from build123d import *

# Parameters (mm, degrees)
SKETCH1_W             = 89.6514
SKETCH1_H             = 226.9314
SKETCH1_R             = 2
HEAT_EXCHANGER_DEPTH  = 0.0686
CONVECTION_FINS_DEPTH = 7.0524
TOP_OVERWRAP_DEPTH    = 0.0686
SIDE_OVERWRAP_DEPTH   = 0.0686


# Read off the part's stored shape, not the designer's step: Mirror1
with BuildPart() as part:
    # Sketch1 → Heat Exchanger (new body)
    with BuildSketch(Plane.XY):
        with Locations((-44.8257, 0)):
            Rectangle(SKETCH1_W, SKETCH1_H)
        with Locations((-83.71996294, -56.7081132)):
            Circle(SKETCH1_R, mode=Mode.SUBTRACT)
        with Locations((-83.71996294, 56.94427919)):
            Circle(SKETCH1_R, mode=Mode.SUBTRACT)
    extrude(amount=HEAT_EXCHANGER_DEPTH)

    # Sketch3 → Convection Fins (add)
    with BuildSketch(Plane.XY):
        Polygon((0, -113.5343), (0, -113.4657), (-89.6514, -113.4657), (-89.6514, 113.4657), (-89.72, 113.4657), (-89.72, -113.5343), align=None)
    extrude(amount=CONVECTION_FINS_DEPTH)

    # Sketch5 → Top Overwrap (add)
    with BuildSketch(Plane(origin=(0, 113.4657, 0), x_dir=(1, 0, 0), z_dir=(0, 1, 0))):
        Polygon((-89.8724, -7.0524), (-89.6514, -7.0524), (-89.6514, -0.0686), (0, -0.0686), (0, 0.1524), (-89.8724, 0.1524), align=None)
    extrude(amount=TOP_OVERWRAP_DEPTH)

    # Sketch7 → Side Overwrap (add)
    with BuildSketch(Plane.XY.offset(7.0524)):
        Polygon((-89.8724, 113.5343), (-89.6514, 113.5343), (-89.6514, -113.4657), (0, -113.4657), (0, -113.6867), (-89.8724, -113.6867), align=None)
    extrude(amount=SIDE_OVERWRAP_DEPTH)

    # Mirror1: part across plane


with BuildPart() as part_1:
    add(part.part)
    add(part.part.mirror(Plane(origin=(0, 0, 0), x_dir=(0, 0, 1), z_dir=(1, 0, 0))))


solid = part_1.part
For this review, take the finished solid that the model builds, in its own axes (mm). Round coordinates to 2 decimals unless told otherwise and drop trailing zeros. Loops run counter-clockwise (first coordinate to the right, second up) from the corner with the lowest first, then second, coordinate; pieces in that order, holes last. Notation, with made-up numbers: (43.25, 6.5) - (71.25, 6.5) arc R31 cw to (71.25, 34.5) - close; hole circle Ø11 at (-10, 4). An arc over 180 degrees is marked (long way). Put each result on its own line as item: value. Start each with the question number.
1. Insertion check: P1, Ø2, axis at x = 35.5, z = 1, coming from the +Y side; P2, Ø3.5, axis at y = -29, z = 2.5, coming from the +X side; P3, Ø3.5, axis at y = -44, z = 3.5, coming from the -X side; P4, Ø4, axis at x = -43, y = 68.5, coming from the -Z side. Each pin has a flat end and moves straight along its axis. Give the tip position at first contact, or say it passes through.
2. Consider section B-B on x = 53. State the section outline as (y, z) points.
3. Consider section C-C on y = 81. State the section outline as (x, z) points, plus the area to 3 significant figures.
4. Consider section A-A on z = 3.5. State the section outline as (x, y) points, plus the area to 3 significant figures.
Result sheet:
1. P1: y = 113.53
1. P2: x = 89.72
1. P3: x = -89.72
1. P4: z = 0
2. outline: (-113.69, 7.05) - (-113.53, 7.05) - (-113.53, 0) - (113.47, 0) - (113.47, -0.15) - (113.53, -0.15) - (113.53, 0.07) - (-113.47, 0.07) - (-113.47, 7.12) - (-113.69, 7.12) - close
3. outline: (-89.87, 7.05) - (-89.72, 7.05) - (-89.72, 0) - (89.72, 0) - (89.72, 7.05) - (89.87, 7.05) - (89.87, 7.12) - (89.65, 7.12) - (89.65, 0.07) - (-89.65, 0.07) - (-89.65, 7.12) - (-89.87, 7.12) - close
3. area: 13.3 mm^2
4. outline: (-89.87, 113.47) - (-89.72, 113.47) - (-89.72, -113.53) - (89.72, -113.53) - (89.72, 113.47) - (89.87, 113.47) - (89.87, 113.53) - (89.65, 113.53) - (89.65, -113.47) - (-89.65, -113.47) - (-89.65, 113.53) - (-89.87, 113.53) - close
4. area: 43.5 mm^2
